Autodesk Inventor part; units mm, degrees
ref_plane "YZ Plane" through (0, 0, 0) normal (1, 0, 0) x (0, 1, 0)
ref_plane "XZ Plane" through (0, 0, 0) normal (0, 1, 0) x (-1, 0, 0)
sketch "Sketch1" plane through (0, 0, 0) normal (1, 0, 0) x (0, 1, 0)
  circle A0 centre (0, 0) radius 3
  dimension "d4" = 6
extrude "Extrusion1" add sketch "Sketch1" along normal blind 370
sketch "Sketch2" plane through (370, 0, 0) normal (1, 0, 0) x (0, 0, -1)
  circle A0 centre (0, 0) radius 2
  dimension "d5" = 4
extrude "Extrusion2" add sketch "Sketch2" along normal blind 4
thread "Thread1"
ref_plane "Work Plane1" through (0, 0, -3) normal (0, 0, 1) x (1, 0, 0)
sketch "Sketch3" plane through (0, 0, -3) normal (0, 0, 1) x (1, 0, 0)
  line L0 (374, 0.5) -> (368, 0.5)
  line L1 (368, 0.5) -> (368, -0.5)
  line L2 (368, -0.5) -> (374, -0.5)
  line L3 (374, -0.5) -> (374, 0.5)
  line L4 (374, 0.5) -> (368, -0.5) construction
  line L5 (368, 0.5) -> (374, -0.5) construction
  line L6 (374, -2) -> (374, 2)
  point P0 (0, 0)
  point P1 (371, 0)
  dimension "d10" = 1
  dimension "d11" = 6
  dimension "d18" = 0
extrude "Extrusion3" cut sketch "Sketch3" along normal blind 1.5
sketch "Sketch4" plane through (0, 0, -3) normal (0, 0, 1) x (1, 0, 0)
  circle A0 centre (360, 0) radius 1
  line L0 (370, -3) -> (370, 3)
  point P0 (0, 0)
  point P1 (370, 0.5)
  point P2 (370, -0.5)
  dimension "d14" = 2
  dimension "d15" = 10
extrude "Extrusion4" cut sketch "Sketch4" along normal up to next
properties part number "Rod"
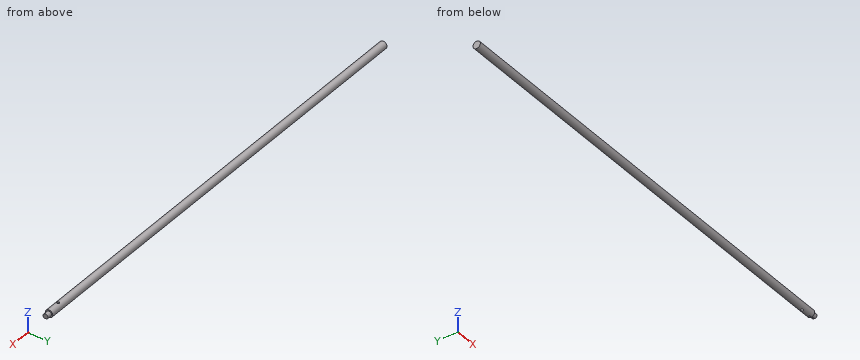
For this review, take the finished solid that the model builds, in its own axes (mm). Give positions to 0.01 mm unless a question says otherwise; leave off trailing zeros. Order: outer loops, then holes, each group sorted by start corner. A loop starts at its lowest first (then second) coordinate and runs counter-clockwise, first axis right, second up. Notation, with made-up numbers: M 77,-10.5 L 126,-10.5 A11 ccw 126,-3.5 Z; hole C 2.5,75 d1. An arc over 180 degrees is marked long. Answer in a Markdown table with one row per item. Add a question column.
(1) For pin 1 (0.7 mm diameter, centred on x = 370, z = -2, fed in from +Y); pin 2 (3 mm diameter, centred on x = 134.5, y = -2, fed in from -Z); pin 3 (2 mm diameter, centred on x = 330, z = -2, fed in from +Y), all flat-tipped, find the tip position at first contact; note any pin that passes through.
(2) Consider section A-A on x = 315.5. State the section outline as (y, z) points, and give its area (3 significant figures).
(3) Wall thickness on probe 1 along X at (y, z) = (0, -0.5); probe 2 along Y at (x, z) = (360, 0); probe 3 along Z at (x, y) = (28, 2.25): over which ranges is each line inside the solid? List them lowest first. Write a range as [from, to].
Evaluation:
| question | item | result |
|---|---|---|
| 1 | pin 1 | stops at y = 2.51 |
| 1 | pin 2 | stops at z = -2.96 |
| 1 | pin 3 | stops at y = 2.83 |
| 2 | outline | C 0,0 d6 |
| 2 | area | 28.3 mm^2 |
| 3 | probe 1 | x = [0, 359], [361, 374] |
| 3 | probe 2 | y = [-3, -1], [1, 3] |
| 3 | probe 3 | z = [-1.98, 1.98] |
